from build123d import *

# Parameters (mm, degrees)
CROQUIS1_R              = 2
CROQUIS1_R_2            = 1.55
SALIENTE_EXTRUIR1_DEPTH = 24
CORTAR_EXTRUIR1_DEPTH   = 20
REDONDEO1_R             = 8
REDONDEO2_R             = 2
REDONDEO5_R             = 2.5
CROQUIS3_R              = 2.2
CORTAR_EXTRUIR2_DEPTH   = 20
CROQUIS4_W              = 1.5
CROQUIS4_H              = 7.2
CORTAR_EXTRUIR3_DEPTH   = 20
SALIENTE_EXTRUIR2_REACH = 43.512
REDONDEO7_R             = 2
CROQUIS6_W              = 7.2
CROQUIS6_H              = 3
CORTAR_EXTRUIR4_DEPTH   = 1.5
REDONDEO8_R             = 3
REDONDEO9_R             = 5
CHAFL_N1_SIZE           = 0.3
CHAFL_N1_SIZE2          = 0.519615242


with BuildPart() as part:
    # Croquis1 → Saliente-Extruir1 (new body)
    with BuildSketch(Plane.XY):
        with BuildLine():
            Line((-5.5, 0), (-5.5, 31.5))
            Line((-5.5, 31.5), (-3, 31.5))
            Line((-3, 31.5), (-3, 20.05))
            Line((-3, 20.05), (2.45, 20.05))
            ThreePointArc((2.45, 20.05), (6.941557686, 15.825516889), (3, 11.08373758))
            Line((3, 11.08373758), (3, 0))
            ThreePointArc((3, 0), (2.121320344, -2.121320344), (0, -3))
            Line((0, -3), (-2.5, -3))
            ThreePointArc((-2.5, -3), (-4.621320344, -2.121320344), (-5.5, 0))
        make_face()
        with Locations((2.45, 15.55)):
            Circle(CROQUIS1_R, mode=Mode.SUBTRACT)
        Circle(CROQUIS1_R_2, mode=Mode.SUBTRACT)
    extrude(amount=SALIENTE_EXTRUIR1_DEPTH)

    # Croquis2 → Cortar-Extruir1 (cut)
    with BuildSketch(Plane.ZY.offset(5.5)):
        Polygon((1.5, -3), (19.7, -3), (19.7, 11), (17.7, 11), (17.7, 23), (1.5, 23), align=None)
    extrude(amount=-CORTAR_EXTRUIR1_DEPTH, mode=Mode.SUBTRACT)

    # Redondeo1
    redondeo1_edges = [part.edges().sort_by_distance(p)[0] for p in [
        (-4.25, 31.5, 0),
        (-4.25, 31.5, 24),
    ]]
    fillet(redondeo1_edges, radius=REDONDEO1_R)

    # Redondeo2
    redondeo2_edges = [part.edges().sort_by_distance(p)[0] for p in [
        (-1.25, 11, 19.7),
        (-4.25, 23, 17.7),
        (-4.25, 23, 1.5),
    ]]
    fillet(redondeo2_edges, radius=REDONDEO2_R - 0.0001)  # a hair under: the kernel refuses the full size

    # Redondeo5
    redondeo5_edges = [part.edges().sort_by_distance(p)[0] for p in [
        (3, 11.08373758, 0.75),
        (-3, 20.05, 20.85),
        (3, 11.08373758, 20.85),
        (-3, 20.05, 0.75),
    ]]
    fillet(redondeo5_edges, radius=REDONDEO5_R)

    # Croquis3 → Cortar-Extruir2 (cut)
    with BuildSketch(Plane.ZY.offset(5.5)):
        with Locations((7.8, 26.4)):
            Circle(CROQUIS3_R)
    extrude(amount=-CORTAR_EXTRUIR2_DEPTH, mode=Mode.SUBTRACT)

    # Croquis4 → Cortar-Extruir3 (cut)
    with BuildSketch(Plane.XZ.offset(-23)):
        with Locations((-4.75, 7.8)):
            Rectangle(CROQUIS4_W, CROQUIS4_H)
    extrude(amount=-CORTAR_EXTRUIR3_DEPTH, mode=Mode.SUBTRACT)

    # Saliente-Extruir2: up to this face of the body (flat: up to its plane)
    saliente_extruir2_end = Plane(part.part.faces().sort_by_distance((-3, 26.79790631, 12.475730365))[0])
    # Croquis5 → Saliente-Extruir2 (add, up to the picked face)
    with BuildSketch(Plane.ZY.offset(5.5), mode=Mode.PRIVATE) as saliente_extruir2_sk1:
        Polygon((0, 23.5), (0, 48.5), (12, 48.5), (12, 30), (4.2, 30), align=None)
    saliente_extruir2_tool1 = split(extrude(saliente_extruir2_sk1.sketch, amount=-SALIENTE_EXTRUIR2_REACH, mode=Mode.PRIVATE), bisect_by=saliente_extruir2_end, keep=Keep.BOTH, mode=Mode.PRIVATE)
    add(saliente_extruir2_tool1.solids().sort_by(Axis((-5.5, 38.588691, 5.733546), (1, 0, 0)))[0])

    # Redondeo7
    redondeo7_edges = [part.edges().sort_by_distance(p)[0] for p in [
        (-4.25, 31.5, 12),
    ]]
    fillet(redondeo7_edges, radius=REDONDEO7_R)

    # Croquis6 → Cortar-Extruir4 (cut)
    with BuildSketch(Plane.ZY.offset(5.5)):
        with Locations((7.8, 30)):
            Rectangle(CROQUIS6_W, CROQUIS6_H)
    extrude(amount=-CORTAR_EXTRUIR4_DEPTH, mode=Mode.SUBTRACT)

    # Redondeo8
    redondeo8_edges = [part.edges().sort_by_distance(p)[0] for p in [
        (-4.75, 31.5, 4.2),
        (-4.75, 31.5, 11.4),
    ]]
    fillet(redondeo8_edges, radius=REDONDEO8_R)

    # Redondeo9
    redondeo9_edges = [part.edges().sort_by_distance(p)[0] for p in [
        (-4.25, 48.5, 12),
        (-4.25, 48.5, 0),
    ]]
    fillet(redondeo9_edges, radius=REDONDEO9_R)

    # Chaflán1
    chafl_n1_edges = [part.edges().sort_by_distance(p)[0] for p in [
        (0.45, 15.55, 24),
    ]]
    chafl_n1_side = [part.faces().sort_by_distance(p)[0] for p in [
        (-0.877926413, 10.141568141, 24),
    ]]
    chamfer(chafl_n1_edges, length=CHAFL_N1_SIZE, length2=CHAFL_N1_SIZE2, reference=chafl_n1_side[0])


solid = part.part
Geometry check sheet. Reference: the model listing, model coordinates, mm. A direction names the side the tool comes from. Give positions to 0.01 mm unless a question says otherwise; leave off trailing zeros. Loops run counter-clockwise (first coordinate to the right, second up) from the corner with the lowest first, then second, coordinate; pieces in that order, holes last.
(1) Set-up check for faces 1 (the cylindrical face through (-0.83, 10.43, 19.1)), 2 (the flat face through (-5, 31.5, 8)), 3 (the flat face through (1, 20.05, 21)), 4 (the flat face through (3, 5, 1)): record each of +Z, -Z, +X, -X, +Y, -Y from which the full face is reachable in a straight line by a thin tool's end or side.
From the geometry:
face 1: +X, -X, -Y
face 2: -X, -Y
face 3: +Z, -Z, +X, +Y
face 4: +Z, -Z, +X, -Y
(2) Section check D-D on y = 27. Record the cut outline in (x, z), then the cut area to 3 significant figures.
From the geometry:
outline: (-5.5, 0) - (-3, 0) - (-3, 5.68) - (-4, 5.68) - (-4, 4.2) - (-5.5, 4.2) - close; (-5.5, 11.4) - (-4, 11.4) - (-4, 9.92) - (-3, 9.92) - (-3, 23.19) - (-5.5, 23.19) - close
area: 43.0 mm2
(3) Section check B-B on y = 15.55. Record the cut outline in (x, z).
From the geometry:
outline: (-5.5, 0) - (0.45, 0) - (0.45, 1.5) - (-5.5, 1.5) - close; (-5.5, 17.7) - (0.45, 17.7) - (0.45, 23.48) - (0.15, 24) - (-5.5, 24) - close; (4.45, 0) - (6.95, 0) - (6.95, 1.5) - (4.45, 1.5) - close; (4.45, 17.7) - (6.95, 17.7) - (6.95, 24) - (4.75, 24) - (4.45, 23.48) - close
(4) Section check C-C on z = 9.25. Record the cut outline in (x, y).
From the geometry:
outline: (-5.5, 31.38) - (-4, 31.38) - (-4, 28.05) - (-3, 28.05) - (-3, 47.97) - (-5.5, 47.97) - close; (-4, 23) - (-3, 23) - (-3, 24.75) - (-4, 24.75) - close
(5) Release check for a two-part mould opening along X. For faces 5 (the flat face through (-3, 33, 9)), 6 (the cylindrical face through (0.715, -1.375, 21.82)), 7 (the flat face through (-1, 16, 17.7)), 8 (the flat face through (-4, 28, 6)) record: released by +X, released by -X, zero draft, split by the parting line, or undercut.
From the geometry:
face 5: released by +X
face 6: undercut
face 7: zero draft
face 8: released by -X
(6) Section check A-A on y = 3. Record the cut outline in (x, z).
From the geometry:
outline: (-5.5, 0) - (3, 0) - (3, 1.5) - (-5.5, 1.5) - close; (-5.5, 19.7) - (3, 19.7) - (3, 24) - (-5.5, 24) - close
(7) Depth check by flat-ended pin: pin 1 Ø1.2 at (x, y) = (-4, 40) entering from +Z; pin 2 Ø1 at (x, z) = (-4, 14.5) entering from +Y; pin 3 Ø5 at (y, z) = (26.4, 7.8) entering from +X. Enter the tip coordinate at first touch or a pass-through.
From the geometry:
pin 1: stops at z = 12
pin 2: stops at y = 31.5
pin 3: stops at x = -3
(8) Thickness scan on L1, parallel to X at y = 15.55, z = 1.1; L2, parallel to X at y = 0, z = 21.95; L3, parallel to Z at x = -4.25, y = 18. Record the ranges inside material, lowest first.
From the geometry:
L1: x = -5.5 to 0.45, 4.45 to 6.95
L2: x = -5.5 to -1.55, 1.55 to 3
L3: z = 0 to 1.5, 17.7 to 24
